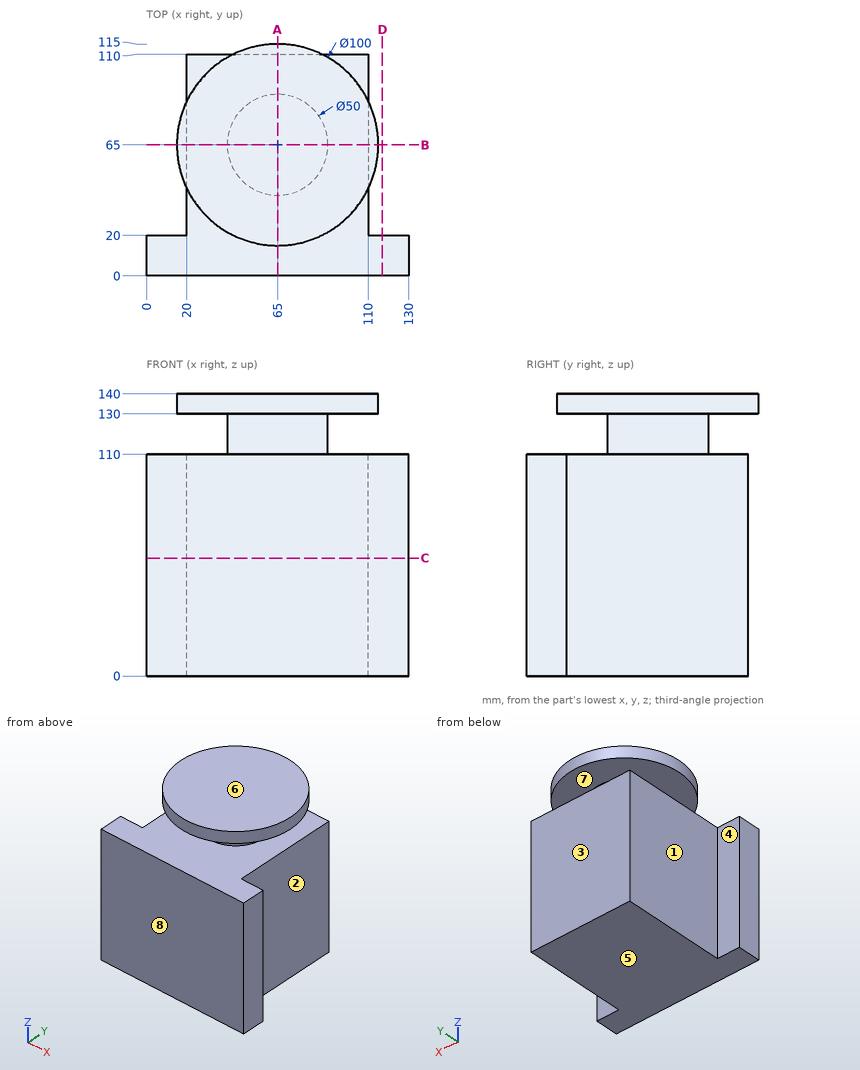
Geometry check sheet. Reference: drawing and pictorial views, mm from the part's lowest x, y, z. A direction names the side the tool comes from. Give positions to 0.01 mm unless a question says otherwise; leave off trailing zeros. Loops run counter-clockwise (first coordinate to the right, second up) from the corner with the lowest first, then second, coordinate; pieces in that order, holes last. Notation, with made-up numbers: M 75.25,-22.75 L 118.25,-22.75 A21 cw 118.25,6.25 Z; hole C 68.5,5 d6. An arc over 180 degrees is marked long. One line per question, with ' | ' between items.
Item 1: Depth check by flat-ended pin: P1, Ø6, axis at x = 14.5, y = 51.5, coming from the -Z side; P2, Ø12, axis at x = 86, z = 57, coming from the +Y side; P3, Ø6, axis at x = 81, z = 113.5, coming from the -Y side. Enter the tip coordinate at first touch or a pass-through.
Completed:
P1: stops at z = 130 | P2: stops at y = 110 | P3: stops at y = 43.65
Item 2: Section check C-C, the plane z = 58.5. Record the cut outline in (x, y).
Completed:
outline: M 0,0 L 130,0 L 130,20 L 110,20 L 110,110 L 20,110 L 20,20 L 0,20 Z
Item 3: Tool access check on the marked faces 1, 2, 3 and 4. Record the directions out of +Z, -Z, +X, -X, +Y, -Y that give a thin tool (end or side, any length) a straight path to the whole face; none if there is none.
Completed:
face 1: -Z, -X, +Y | face 2: -Z, +X, +Y | face 3: -Z, +X, -X, +Y | face 4: +Z, -Z, -X, +Y
Item 4: Thickness scan on line 1 (Z direction, x = 75.5, y = 32.5); line 2 (X direction, y = 81, z = 87.5); line 3 (Y direction, x = 33, z = 64.5). Record the ranges inside material, lowest first. Write a range as [from, to].
Completed:
line 1: z = [0, 110], [130, 140] | line 2: x = [20, 110] | line 3: y = [0, 110]
Item 5: Section check A-A, the plane x = 65. Record the cut outline in (y, z).
Completed:
outline: M 0,0 L 110,0 L 110,110 L 90,110 L 90,130 L 115,130 L 115,140 L 15,140 L 15,130 L 40,130 L 40,110 L 0,110 Z
Item 6: Section check D-D, the plane x = 117. Record the cut outline in (y, z).
Completed:
outline: M 0,0 L 20,0 L 20,110 L 0,110 Z
Item 7: Section check B-B, the plane y = 65. Record the cut outline in (x, z), plus the area to 3 significant figures.
Completed:
outline: M 15,130 L 40,130 L 40,110 L 20,110 L 20,0 L 110,0 L 110,110 L 90,110 L 90,130 L 115,130 L 115,140 L 15,140 Z | area: 11,900 mm^2
Item 8: Draft check along Z on the marked faces 5, 6, 7 and 8. Enter one of: +Z half, -Z half, draft (parallel to the pull), parting line (faces both ways), or undercut.
Completed:
face 5: -Z half | face 6: +Z half | face 7: undercut | face 8: draft
